```python
from build123d import *

# Parameters (mm, degrees)
F0_W     = 114.3
F0_H     = 12.7
F1_DEPTH = 21.59
F3_DEPTH = 25.4
F2_R     = 3.175
F4_DEPTH = 25.4


with BuildPart() as f1:
    # F0 (on Front) → F1 (new body)
    with BuildSketch(Plane.XZ):
        with Locations((57.15, 6.35)):
            Rectangle(F0_W, F0_H)
    extrude(amount=F1_DEPTH)

    # F2 (on face) → F3 (join)
    with BuildSketch(Plane.XY.offset(12.7)):
        with BuildLine():
            ThreePointArc((6.985, -7.62), (3.81, -4.445), (0.635, -7.62))
            ThreePointArc((0.635, -7.62), (3.81, -10.795), (6.985, -7.62))
        make_face()
    extrude(amount=F3_DEPTH)

    # F2 (on face) → F4 (join)
    with BuildSketch(Plane.XY.offset(12.7)):
        with Locations((110.49, -7.62)):
            Circle(F2_R)
    extrude(amount=F4_DEPTH)


solid = f1.part
```
Can you work these out from the model? Positions are in its coordinate system, mm. A direction names the side the tool comes from. Coordinates: 2 decimals unless noted, no trailing zeros. Order: outer loops, then holes, each group sorted by start corner. A loop starts at its lowest first (then second) coordinate and runs counter-clockwise, first axis right, second up. Notation, with made-up numbers: (62, 70) -> (118, 70) arc R25 cw to (118, 94) -> close; hole circle Ø7 at (-28.75, 14.5). An arc over 180 degrees is marked (long way). Write each question's results on one line, items separated by ' | '.
Item 1: I want a section at D-D, the plane x = 91. Write out the boundary of the cut face in (y, z).
Results are:
outline: (-21.59, 0) -> (0, 0) -> (0, 12.7) -> (-21.59, 12.7) -> close
Item 2: If I drill on line 1 along Z through (x, y) = (5, -20.5); line 2 along X through (y, z) = (-10, 13.5); line 3 along X through (y, z) = (-8.25, 31.5), over which ranges is the centre line in solid material (lowest first)?
Results are:
line 1: 0 to 12.7 | line 2: 1.71 to 5.91, 108.39 to 112.59 | line 3: 0.7 to 6.92, 107.38 to 113.6
Item 3: I want a section at A-A, the plane x = 110.49. Write out the boundary of the cut face in (y, z) (3 decimals).
Results are:
outline: (-21.59, 0) -> (0, 0) -> (0, 12.7) -> (-4.445, 12.7) -> (-4.445, 38.1) -> (-10.795, 38.1) -> (-10.795, 12.7) -> (-21.59, 12.7) -> close
Item 4: I want a section at B-B, the plane y = -7.62. Write out the boundary of the cut face in (x, z) (3 decimals), then the cut area to 3 significant figures.
Results are:
outline: (0, 0) -> (114.3, 0) -> (114.3, 12.7) -> (113.665, 12.7) -> (113.665, 38.1) -> (107.315, 38.1) -> (107.315, 12.7) -> (6.985, 12.7) -> (6.985, 38.1) -> (0.635, 38.1) -> (0.635, 12.7) -> (0, 12.7) -> close | area: 1,770 mm²
Item 5: Which directions (+Z, -Z, +X, -X, +Y, -Y) give clear straight access to the entire face, cutting with the end or side of a thin tool? Please do faces 4 (the face through (56, -11, 0)), 5 (the face through (113.52, -6.67, 25.22)).
Results are:
face 4: -Z, +X, -X, +Y, -Y | face 5: +Z
Item 6: I want a section at C-C, the plane z = 32. Write out the boundary of the cut face in (x, y) (3 decimals), then the cut area to 3 significant figures.
Results are:
outline: circle Ø6.35 at (3.81, -7.62); circle Ø6.35 at (110.49, -7.62) | area: 63.3 mm²
Item 7: If we mould it in two halves opening along X, with no side actions, what happens to faces 1 (the face through (56, -11, 12.7)), 2 (the face through (0, -11, 6)), 3 (the face through (4, -8, 38.1))? For each: +X half, -X half, draft (parallel to the pull), parting line (faces both ways), or undercut.
Results are:
face 1: undercut | face 2: -X half | face 3: draft
Item 8: I'm going to push flat-ended pins straight in: pin 1 Ø6.5 at (x, y) = (47, -11) entering from +Z; pin 2 Ø10 at (y, z) = (-5, 31.5) entering from -X (3 decimals). Where does each tip first touch, or does it pass through?
Results are:
pin 1: z = 12.7 | pin 2: x = 0.635
